```python
from build123d import *

# Parameters (mm, degrees)
BOSS_EXTRUDE2_DEPTH     = 26
SHELL3_T                = -5
SKETCH2_W               = 3
SKETCH2_H               = 20
BOSS_EXTRUDE3_DEPTH     = 6
BOSS_EXTRUDE4_DEPTH     = 7
BOSS_EXTRUDE4_TAPER     = 1
BOSS_EXTRUDE5_START     = -7.07
BOSS_EXTRUDE5_OUTLINE_W = 12
BOSS_EXTRUDE5_OUTLINE_H = 3
BOSS_EXTRUDE5_DEPTH     = 13.778752476
SKETCH7_W               = 4
SKETCH7_H               = 7.778752476
CUT_EXTRUDE1_DEPTH      = 3
CUT_EXTRUDE5_DEPTH      = 3
SKETCH8_W               = 2
SKETCH8_H               = 6.204571956
BOSS_EXTRUDE6_DEPTH     = 3
BOSS_EXTRUDE6_DRAFT     = -14
SKETCH10_W              = 10
SKETCH10_H              = 3
CUT_EXTRUDE2_DEPTH      = 3
CHAMFER2_SIZE           = 1.5
CHAMFER2_SIZE_2         = 1.061054559
FILLET7_R               = 1.5


# Read off the part's stored shape, not the designer's step: Boss-Extrude5
with BuildPart() as part:
    # Sketch1 → Boss-Extrude2 (new, symmetric)
    with BuildSketch(Plane(origin=(0, 0, 0), x_dir=(0, 0, -1), z_dir=(1, 0, 0))):
        Polygon((-7.07, 6.681327836), (-7.07, -7.07), (7.452430332, -7.07), align=None)
    extrude(amount=BOSS_EXTRUDE2_DEPTH, both=True)

    # Shell3
    shell3_openings = [part.faces().sort_by_distance(p)[0] for p in [
        (0, -0.194336082, 7.07),
        (0, -7.07, -0.191215166),
    ]]
    offset(amount=SHELL3_T, openings=shell3_openings, kind=Kind.INTERSECTION)

    # Sketch2 → Boss-Extrude3 (add)
    with BuildSketch(Plane(origin=(0, -0.006998714, 0.006627101), x_dir=(1, 0, 0), z_dir=(0, 0.7261215165867746, -0.6875663918122543))):
        with Locations((-24.5, 0.272464405)):
            Rectangle(SKETCH2_W, SKETCH2_H)
    boss_extrude3 = extrude(amount=BOSS_EXTRUDE3_DEPTH)

    # Sketch3 → Boss-Extrude4 (add)
    with BuildSketch(Plane(origin=(-23, 0, 0), x_dir=(0, 0, -1), z_dir=(1, 0, 0))):
        Polygon((-5.007300825, 8.859692386), (0.075549792, 4.046727643), (2.138248967, 6.225092193), (-2.944601649, 11.038056936), align=None)
    boss_extrude4 = extrude(amount=BOSS_EXTRUDE4_DEPTH, taper=BOSS_EXTRUDE4_TAPER)

    # Boss-Extrude5 outline → Boss-Extrude5 (add)
    with BuildSketch(Plane(origin=(0, 0, 0), x_dir=(1, 0, 0), z_dir=(0, 1, 0)).offset(BOSS_EXTRUDE5_START)):
        with Locations((-27, -8.57)):
            Rectangle(BOSS_EXTRUDE5_OUTLINE_W, BOSS_EXTRUDE5_OUTLINE_H)
    boss_extrude5 = extrude(amount=BOSS_EXTRUDE5_DEPTH)

    # Sketch7 → Cut-Extrude1 (cut)
    with BuildSketch(Plane(origin=(0, 0, 7.07), x_dir=(-1, 0, 0), z_dir=(0, 0, -1))):
        with Locations((28, -0.180623762)):
            Rectangle(SKETCH7_W, SKETCH7_H)
    cut_extrude1 = extrude(amount=-CUT_EXTRUDE1_DEPTH, mode=Mode.SUBTRACT)

    # Sketch11 → Cut-Extrude5 (cut)
    with BuildSketch(Plane(origin=(0.097524812, 4.056980848, -3.841565936), x_dir=(0.9998476951563913, -0.012672567830329124, 0.011999688122524015), z_dir=(0.017452406437283557, 0.72601092476275, -0.6874616721204788))):
        with BuildLine():
            ThreePointArc((-16.099976916, -9.605350141), (-20.470201884, -7.075920319), (-23.038834329, -2.72862129))
            add(Edge.make_bspline(
                [(-23.038834329, -2.72862129), (-20.964785252, -1.12213519), (-16.845095332, -0.866613762), (-13.311050846, -5.432002143), (-14.677947992, -8.654526842), (-16.099976916, -9.605350141)],
                knots=[0, 0, 0, 0, 0.462245197, 0.666716807, 1, 1, 1, 1], degree=3))
        make_face()
    cut_extrude5 = extrude(amount=-CUT_EXTRUDE5_DEPTH, mode=Mode.SUBTRACT)

    # Mirror4: Boss-Extrude3, Boss-Extrude4, Boss-Extrude5, Cut-Extrude1, Cut-Extrude5 across plane
    add(boss_extrude3.mirror(Plane(origin=(0, 0, 0), x_dir=(0, 0, 1), z_dir=(1, 0, 0))))
    add(boss_extrude4.mirror(Plane(origin=(0, 0, 0), x_dir=(0, 0, 1), z_dir=(1, 0, 0))))
    add(boss_extrude5.mirror(Plane(origin=(0, 0, 0), x_dir=(0, 0, 1), z_dir=(1, 0, 0))))
    add(cut_extrude1.mirror(Plane(origin=(0, 0, 0), x_dir=(0, 0, 1), z_dir=(1, 0, 0))), mode=Mode.SUBTRACT)
    add(cut_extrude5.mirror(Plane(origin=(0, 0, 0), x_dir=(0, 0, 1), z_dir=(1, 0, 0))), mode=Mode.SUBTRACT)


with BuildPart() as boss_extrude6_tool:
    # Sketch8 → Boss-Extrude6 (with draft: the straight prism first)
    with BuildSketch(Plane.XY.offset(7.07)):
        with Locations((0, 2.897714022)):
            Rectangle(SKETCH8_W, SKETCH8_H)
    extrude(amount=BOSS_EXTRUDE6_DEPTH)
    # Boss-Extrude6: the draft: its side faces are tilted about the plane it starts from
    boss_extrude6_sides = [boss_extrude6_tool.faces().sort_by_distance(p)[0] for p in [
        (0, -0.204571956, 8.57),
        (1, 2.897714022, 8.57),
        (0, 6, 8.57),
        (-1, 2.897714022, 8.57),
    ]]
    draft(boss_extrude6_sides, Plane.XY.offset(7.07), BOSS_EXTRUDE6_DRAFT)


with BuildPart() as part_1:
    add(part.part)

    # Boss-Extrude6: add boss_extrude6_tool
    add(boss_extrude6_tool.part)

    # Sketch10 → Cut-Extrude2 (cut)
    with BuildSketch(Plane(origin=(0, -0.006998714, 0.006627101), x_dir=(1, 0, 0), z_dir=(0, 0.7261215165867746, -0.6875663918122543))):
        with Locations((0, 8.772464405)):
            Rectangle(SKETCH10_W, SKETCH10_H)
    extrude(amount=-CUT_EXTRUDE2_DEPTH, mode=Mode.SUBTRACT)

    # Chamfer2
    # the kernel refuses this chamfer: 1.5, 1.061054559 mm, written as the material it takes off along each edge
    with BuildSketch(Plane(origin=(21, 6.681327836, 7.07), x_dir=(0, -0.6673410869627874, -0.7447522229918655), z_dir=(-1, 0, 0))) as chamfer2_piece_1_section:
        Polygon((CHAMFER2_SIZE * 0.999621916911, CHAMFER2_SIZE * 0.0274958766106), (CHAMFER2_SIZE_2 * 0.667341086869, CHAMFER2_SIZE_2 * 0.744752222888), (0, 0), align=None)
    chamfer2_piece_1 = extrude(amount=45.857524482, mode=Mode.PRIVATE)
    chamfer2_piece_1 = split(chamfer2_piece_1, bisect_by=Plane(origin=(1.484835195, 5.763736447, 9.014567757), z_dir=(0.9702957262759965, 0, -0.24192189559966784)), keep=Keep.TOP, mode=Mode.PRIVATE)
    add(chamfer2_piece_1, mode=Mode.SUBTRACT)
    with BuildSketch(Plane(origin=(24.857524482, 6.681327836, 7.07), x_dir=(0, -0.6673410869627874, -0.7447522229918655), z_dir=(-1, 0, 0))) as chamfer2_piece_2_section:
        Polygon((CHAMFER2_SIZE * 0.999621916911, CHAMFER2_SIZE * 0.0274958766106), (CHAMFER2_SIZE_2 * 0.667341086869, CHAMFER2_SIZE_2 * 0.744752222888), (0, 0), align=None)
    chamfer2_piece_2 = extrude(amount=45.857524482, mode=Mode.PRIVATE)
    chamfer2_piece_2 = split(chamfer2_piece_2, bisect_by=Plane(origin=(-1.484835195, 5.763736447, 9.014567757), z_dir=(-0.9702957262759965, 0, -0.24192189559966784)), keep=Keep.TOP, mode=Mode.PRIVATE)
    add(chamfer2_piece_2, mode=Mode.SUBTRACT)
    with BuildSketch(Plane(origin=(24.857524482, 6.681327836, 7.07), x_dir=(0, -0.6673410869627874, -0.7447522229918655), z_dir=(-1, 0, 0))) as chamfer2_piece_3_section:
        Polygon((CHAMFER2_SIZE * 0.999621916911, CHAMFER2_SIZE * 0.0274958766106), (CHAMFER2_SIZE_2 * 0.667341086869, CHAMFER2_SIZE_2 * 0.744752222888), (0, 0), align=None)
    chamfer2_piece_3 = extrude(amount=49.715048964, mode=Mode.PRIVATE)
    chamfer2_piece_3 = split(chamfer2_piece_3, bisect_by=Plane(origin=(0.868426691, 6.154537231, 6.542288281), z_dir=(-0.9702957262759965, 0, 0.24192189559966784)), keep=Keep.TOP, mode=Mode.PRIVATE)
    chamfer2_piece_3 = split(chamfer2_piece_3, bisect_by=Plane(origin=(0, 5.935997372, 6.81329948), z_dir=(0, 0.9702957262759965, -0.24192189559966784)), keep=Keep.TOP, mode=Mode.PRIVATE)
    chamfer2_piece_3 = split(chamfer2_piece_3, bisect_by=Plane(origin=(-0.868426691, 6.154537231, 6.542288281), z_dir=(0.9702957262759965, 0, 0.24192189559966784)), keep=Keep.TOP, mode=Mode.PRIVATE)
    add(chamfer2_piece_3, mode=Mode.SUBTRACT)
    with BuildSketch(Plane(origin=(23, -7.07, -7.452430332), x_dir=(0, 0.7275099269437866, 0.6860971550722583), z_dir=(-1, 0, 0)), Plane(origin=(-1.142475518, -7.07, -7.452430332), x_dir=(0, 0.7275099269437866, 0.6860971550722583), z_dir=(-1, 0, 0))) as chamfer2_piece_4:
        Polygon((CHAMFER2_SIZE_2 * 0.998401282104, -CHAMFER2_SIZE_2 * 0.0565232661308), (CHAMFER2_SIZE * 0.686097155072, -CHAMFER2_SIZE * 0.727509926944), (0, 0), align=None)
    extrude(amount=21.857524482, mode=Mode.SUBTRACT)

    # Fillet7
    # the kernel refuses this fillet: 1.5 mm, written as the material it takes off along each edge
    with BuildSketch(Plane(origin=(21, 5.620273277, 7.07), x_dir=(0, 0.02726259017777431, -0.9996283065103743), z_dir=(-1, 0, 0))) as fillet7_piece_1_section:
        with BuildLine():
            CenterArc((1.460922015, 1.453310189), FILLET7_R, 181.562224917, 74.10480975)
            Line((-0.038520445, 1.412416304), (-0.068509294, 1.411598426))
            Line((-0.068509294, 1.411598426), (-0.029988849, -0.000817878))
            Line((-0.029988849, -0.000817878), (0, -0.03))
            ThreePointArc((0, -0.03), (0.544793634, -0.03), (1.082160572, -0.029066204))
            Line((1.082160572, -0.029066204), (1.089587267, 0))
        make_face()
    fillet7_piece_1 = extrude(amount=23.532353712, mode=Mode.PRIVATE)
    fillet7_piece_1 = split(fillet7_piece_1, bisect_by=Plane(origin=(1.518643203, 5.295979724, 9.15016427), z_dir=(0.9702957262759188, 0, -0.24192189559997973)), keep=Keep.TOP, mode=Mode.PRIVATE)
    add(fillet7_piece_1, mode=Mode.SUBTRACT)
    with BuildSketch(Plane(origin=(21, 5.620273277, 7.07), x_dir=(0, 0.02726259017777431, -0.9996283065103743), z_dir=(-1, 0, 0))) as fillet7_piece_2_section:
        with BuildLine():
            CenterArc((1.460922015, 1.453310189), FILLET7_R, 181.562224917, 74.10480975)
            Line((-0.038520445, 1.412416304), (-0.068509294, 1.411598426))
            Line((-0.068509294, 1.411598426), (-0.029988849, -0.000817878))
            Line((-0.029988849, -0.000817878), (0, -0.03))
            ThreePointArc((0, -0.03), (0.544793634, -0.03), (1.082160572, -0.029066204))
            Line((1.082160572, -0.029066204), (1.089587267, 0))
        make_face()
    fillet7_piece_2 = extrude(amount=23.532353712, mode=Mode.PRIVATE)
    fillet7_piece_2 = split(fillet7_piece_2, bisect_by=Plane(origin=(-0.975981109, 5.302873869, 6.97366549), z_dir=(-0.9702957262759188, 0, -0.24192189559997973)), keep=Keep.TOP, mode=Mode.PRIVATE)
    add(fillet7_piece_2, mode=Mode.SUBTRACT)
    with BuildSketch(Plane(origin=(2.532353712, 5.620273277, 7.07), x_dir=(0, 0.02726259017777401, -0.9996283065103743), z_dir=(-1, 0, 0))) as fillet7_piece_3_section:
        with BuildLine():
            CenterArc((1.460922015, 1.453310189), FILLET7_R, 181.562224917, 74.10480975)
            Line((-0.038520445, 1.412416304), (-0.068509294, 1.411598426))
            Line((-0.068509294, 1.411598426), (-0.029988849, -0.000817878))
            Line((-0.029988849, -0.000817878), (0, -0.03))
            ThreePointArc((0, -0.03), (0.544793634, -0.03), (1.082160572, -0.029066204))
            Line((1.082160572, -0.029066204), (1.089587267, 0))
        make_face()
    fillet7_piece_3 = extrude(amount=23.532353712, mode=Mode.PRIVATE)
    fillet7_piece_3 = split(fillet7_piece_3, bisect_by=Plane(origin=(0.975981109, 5.302873869, 6.97366549), z_dir=(0.9702957262759188, 0, -0.24192189559997973)), keep=Keep.TOP, mode=Mode.PRIVATE)
    add(fillet7_piece_3, mode=Mode.SUBTRACT)
    with BuildSketch(Plane(origin=(2.532353712, 5.620273277, 7.07), x_dir=(0, 0.02726259017777401, -0.9996283065103743), z_dir=(-1, 0, 0))) as fillet7_piece_4_section:
        with BuildLine():
            CenterArc((1.460922015, 1.453310189), FILLET7_R, 181.562224917, 74.10480975)
            Line((-0.038520445, 1.412416304), (-0.068509294, 1.411598426))
            Line((-0.068509294, 1.411598426), (-0.029988849, -0.000817878))
            Line((-0.029988849, -0.000817878), (0, -0.03))
            ThreePointArc((0, -0.03), (0.544793634, -0.03), (1.082160572, -0.029066204))
            Line((1.082160572, -0.029066204), (1.089587267, 0))
        make_face()
    fillet7_piece_4 = extrude(amount=23.532353712, mode=Mode.PRIVATE)
    fillet7_piece_4 = split(fillet7_piece_4, bisect_by=Plane(origin=(-1.518643203, 5.295979724, 9.15016427), z_dir=(-0.9702957262759188, 0, -0.24192189559997973)), keep=Keep.TOP, mode=Mode.PRIVATE)
    add(fillet7_piece_4, mode=Mode.SUBTRACT)
    with BuildSketch(Plane(origin=(-21, -7.07, -0.180405318), x_dir=(0, 0, -1), z_dir=(1, 0, 0))) as fillet7_piece_5:
        with BuildLine():
            CenterArc((FILLET7_R * 0.398330236432, FILLET7_R), FILLET7_R, 226.562224917, 43.437775083)
            Line((-FILLET7_R * 0.28923615538, FILLET7_R * 0.273878483413), (-FILLET7_R * 0.302987483217, FILLET7_R * 0.259356053081))
            Line((-FILLET7_R * 0.302987483217, FILLET7_R * 0.259356053081), (-FILLET7_R * 0.00796660472864, -FILLET7_R * 0.02))
            Line((-FILLET7_R * 0.00796660472864, -FILLET7_R * 0.02), (FILLET7_R * 0.398330236432, -FILLET7_R * 0.02))
            Line((FILLET7_R * 0.398330236432, -FILLET7_R * 0.02), (FILLET7_R * 0.398330236432, 0))
        make_face()
    extrude(amount=42, mode=Mode.SUBTRACT)
    with BuildSketch(Plane(origin=(23, -6.340454545, -6.681975786), x_dir=(0, 0.6875663918122538, 0.7261215165867753), z_dir=(-1, 0, 0)), Plane(origin=(-1.367407216, -6.340454545, -6.681975786), x_dir=(0, 0.6875663918122543, 0.7261215165867746), z_dir=(-1, 0, 0))) as fillet7_piece_6:
        with BuildLine():
            CenterArc((1.453037114, -1.5), FILLET7_R, 90, 71.794047616)
            Line((0.028127716, -1.031349588), (-0.000370472, -1.021976579))
            ThreePointArc((-0.000370472, -1.021976579), (-0.015924991, -0.516492672), (-0.029988849, -0.000817878))
            Line((-0.029988849, -0.000817878), (0, 0.03))
            Line((0, 0.03), (1.453037114, 0.03))
            Line((1.453037114, 0.03), (1.453037114, 0))
        make_face()
    extrude(amount=21.632592784, mode=Mode.SUBTRACT)


solid = part_1.part
```
Read the model definition and answer for the solid it produces. Units are mm, in the model's axes. A direction names the side the tool comes from. Give positions to 0.01 mm unless a question says otherwise; leave off trailing zeros. Write each loop counter-clockwise with the first axis right and the second up, starting at its lowest first coordinate (ties: lowest second). Pieces come first, ordered by that corner, then holes. Notation, with made-up numbers: (-23, -9) - (28, -9) arc R21 cw to (28, 24) - close; hole circle Ø1 at (85, 24.25). An arc over 180 degrees is marked (long way). Write item = value, one per line. Start each with the question number.
Item 1: Find section B-B (y = 0.5). Give the vertices of the cut face in (x, z), then the cut area to 3 significant figures.
Item 2: A tool of negligible diameter and unlimited length cuts with its end or side. For faces 1 (the flat face through (-5, -6, -5)), 2 (the flat face through (27, 6.709, 9)), 3 (the cylindrical face through (-13.874, -6.14, -6.067)), from which of +Z, -Z, +X, -X, +Y, -Y can it reach the whole face along a straight path? Write none if from no direction.
Item 3: Find the intervals of material crossed by probe 1 along X at (y, z) = (-5, 7.5); probe 2 along X at (y, z) = (0, -5.25); probe 3 along X at (y, z) = (-4.75, -3.5), in increasing order. Write a range as [from, to].
Item 4: Each of these flat-tipped pins is pushed along its axis until it touches: P1, Ø2, axis at x = -13.5, y = 1.5, coming from the +Z side; P2, Ø5, axis at y = -1, z = -2, coming from the -X side; P3, Ø1, axis at x = -10, z = 0, coming from the -Y side. Where does it stop, or does it pass through?
Item 5: Find section D-D (z = -10). Give the vertices of the cut face in (x, y).
Item 6: Find section A-A (x = 27.5). Give the vertices of the cut face in (y, z), then the cut area to 3 significant figures.
Item 7: The mould has two halves that part along Y. Classify faces 4 (the flat face through (30, 0, 9)), 5 (the flat face through (24.52, -4.92, -9.49)), 6 (the flat face through (-27, 6.709, 9)): +Y half, -Y half, draft (parallel to the pull), parting line (faces both ways), or undercut.
Item 8: Find section C-C (z = 7.75). Give the vertices of the cut face in (x, y).
Response:
q1.outline = (-33, 7.07) - (-30, 7.07) - (-30, 10.07) - (-33, 10.07) - close; (-26, -8.18) - (-23, -8.18) - (-23, 0.54) - (23, 0.54) - (23, -8.18) - (26, -8.18) - (26, 10.07) - (21, 10.07) - (21, 7.07) - (1, 7.07) - (1.75, 10.07) - (-1.75, 10.07) - (-1, 7.07) - (-21, 7.07) - (-21, 10.07) - (-26, 10.07) - close; (30, 7.07) - (33, 7.07) - (33, 10.07) - (30, 10.07) - close
q1.area = 448 mm²
q2.face_1 = -Z, -Y
q2.face_2 = +Z, +X, -X, +Y
q2.face_3 = -Z
q3.probe_1 = [-33, -21], [21, 33]
q3.probe_2 = [-26, -23], [23, 26]
q3.probe_3 = [-26, 26]
q4.P1 = 7.07
q4.P2 = -26
q4.P3 = -7.04
q5.outline = (-26, -4.38) - (-23, -4.38) - (-23, -1.22) - (-26, -1.22) - close; (23, -4.38) - (26, -4.38) - (26, -1.22) - (23, -1.22) - close
q6.outline = (-7.07, 7.07) - (-4.07, 7.07) - (-4.07, 10.07) - (-7.07, 10.07) - close; (3.71, 7.07) - (6.71, 7.07) - (6.71, 10.07) - (3.71, 10.07) - close
q6.area = 18.0 mm²
q7.face_4 = undercut
q7.face_5 = -Y half
q7.face_6 = +Y half
q8.outline = (-33, -7.07) - (-21, -7.07) - (-21, 6.71) - (-33, 6.71) - close; (-1.17, -0.37) - (1.17, -0.37) - (1.17, 6.17) - (-1.17, 6.17) - close; (21, -7.07) - (33, -7.07) - (33, 6.71) - (21, 6.71) - close; hole (-30, -4.07) - (-26, -4.07) - (-26, 3.71) - (-30, 3.71) - close; hole (26, -4.07) - (30, -4.07) - (30, 3.71) - (26, 3.71) - close
